from build123d import *

# Parameters (mm, degrees)
EXTRUDE_1_DEPTH     = 5
SKETCH_3_R          = 12
EXTRUDE_2_DEPTH     = 5
SKETCH_4_R          = 4
CUT_EXTRUDE_1_DEPTH = 11
SKETCH_6_R          = 2.5
CUT_EXTRUDE_2_DEPTH = 11


with BuildPart() as part:
    # 草图1 → 凸台-拉伸1 (new body)
    with BuildSketch(Plane(origin=(0, 0, 0), x_dir=(1, 0, 0), z_dir=(0, 1, 0))):
        with BuildLine():
            Line((-5.25, 10.790620927), (-18.1875, 4.496092053))
            ThreePointArc((-18.1875, 4.496092053), (-21, 0), (-18.1875, -4.496092053))
            Line((-18.1875, -4.496092053), (-5.25, -10.790620927))
            ThreePointArc((-5.25, -10.790620927), (0, -12), (5.25, -10.790620927))
            Line((5.25, -10.790620927), (18.1875, -4.496092053))
            ThreePointArc((18.1875, -4.496092053), (21, 0), (18.1875, 4.496092053))
            Line((18.1875, 4.496092053), (5.25, 10.790620927))
            ThreePointArc((5.25, 10.790620927), (0, 12), (-5.25, 10.790620927))
        make_face()
    extrude(amount=EXTRUDE_1_DEPTH)

    # 草图3 → 凸台-拉伸2 (add)
    with BuildSketch(Plane(origin=(0, 5, 0), x_dir=(1, 0, 0), z_dir=(0, 1, 0))):
        Circle(SKETCH_3_R)
    extrude(amount=EXTRUDE_2_DEPTH)

    # 草图4 → 切除-拉伸1 (cut, through all)
    with BuildSketch(Plane(origin=(0, 10, 0), x_dir=(1, 0, 0), z_dir=(0, 1, 0))):
        Circle(SKETCH_4_R)
    extrude(amount=-CUT_EXTRUDE_1_DEPTH, mode=Mode.SUBTRACT)

    # 草图6 → 切除-拉伸2 (cut, through all)
    with BuildSketch(Plane.XZ):
        with Locations((-16, 0)):
            Circle(SKETCH_6_R)
        with Locations((16, 0)):
            Circle(SKETCH_6_R)
    extrude(amount=-CUT_EXTRUDE_2_DEPTH, mode=Mode.SUBTRACT)


solid = part.part
Check sheet for the modelled part. Datum: model origin and axes. Units: mm. A direction names the side the tool comes from. Round coordinates to 2 decimals unless told otherwise and drop trailing zeros. Loops run counter-clockwise (first coordinate to the right, second up) from the corner with the lowest first, then second, coordinate; pieces in that order, holes last. Notation, with made-up numbers: (16.25, -19) -> (21.25, -19) arc R15 cw to (21.25, 1) -> close; hole circle Ø5 at (-26, 71). An arc over 180 degrees is marked (long way). Put each result on its own line as item: value. Start each with the question number.
1. Section check C-C (z = 0). Enter the section's corners in (x, y), plus the area to 3 significant figures.
2. Draft check along Z on faces 1 (the face through (-0.867, 5.07, 3.905)), 2 (the face through (13, 5, -1)), 3 (the face through (21, 2, 0)). Enter one of: +Z half, -Z half, draft (parallel to the pull), parting line (faces both ways), or undercut.
3. Section check B-B (y = 2.25). Enter the section's corners in (x, z).
4. Gauge pin test, flat ends, axial feed: pin 1 (1.5 mm diameter, centred on y = 5, z = 9, fed in from +X); pin 2 (6.5 mm diameter, centred on x = -16, z = 0, fed in from -Y); pin 3 (10 mm diameter, centred on x = -16, z = -6.5, fed in from +Y); pin 4 (3 mm diameter, centred on x = 12.5, y = 5.5, fed in from -Z). Record the tip position at first contact, or that the pin passes through.
5. Scan lines: probe 1 along X at (y, z) = (6.75, 0); probe 2 along X at (y, z) = (3, 1); probe 3 along Y at (x, z) = (-19, -1). Record each from-to range of solid material in increasing order.
6. Section check A-A (x = 0). Enter the section's corners in (y, z).
7. Access from +Z, -Z, +X, -X, +Y, -Y to the whole of each face (thin tool, end or side, straight path). Record for faces 4 (the face through (-11.81, 2.46, 7.6)), 5 (the face through (-14, 5, 2)).
8. Section check D-D (y = 5.75). Enter the section's corners in (x, z), plus the area to 3 significant figures.
Findings:
1. outline: (-21, 0) -> (-18.5, 0) -> (-18.5, 5) -> (-21, 5) -> close; (-13.5, 0) -> (-4, 0) -> (-4, 10) -> (-12, 10) -> (-12, 5) -> (-13.5, 5) -> close; (4, 0) -> (13.5, 0) -> (13.5, 5) -> (12, 5) -> (12, 10) -> (4, 10) -> close; (18.5, 0) -> (21, 0) -> (21, 5) -> (18.5, 5) -> close
1. area: 200 mm^2
2. face 1: undercut
2. face 2: draft
2. face 3: parting line
3. outline: (-18.19, -4.5) -> (-5.25, -10.79) arc R12 ccw to (5.25, -10.79) -> (18.19, -4.5) arc R5 ccw to (18.19, 4.5) -> (5.25, 10.79) arc R12 ccw to (-5.25, 10.79) -> (-18.19, 4.5) arc R5 ccw to start; hole circle Ø5 at (-16, 0); hole circle Ø8 at (0, 0); hole circle Ø5 at (16, 0)
4. pin 1: stops at x = 10.47
4. pin 2: stops at y = 0
4. pin 3: stops at y = 5
4. pin 4: stops at z = -7.95
5. probe 1: x = -12 to -4, 4 to 12
5. probe 2: x = -20.9 to -18.29, -13.71 to -3.87, 3.87 to 13.71, 18.29 to 20.9
5. probe 3: y = 0 to 5
6. outline: (0, -12) -> (10, -12) -> (10, -4) -> (0, -4) -> close; (0, 4) -> (10, 4) -> (10, 12) -> (0, 12) -> close
7. face 4: +Z, -X, +Y, -Y
7. face 5: -X, +Y
8. outline: circle Ø24 at (0, 0); hole circle Ø8 at (0, 0)
8. area: 402 mm^2
